For this review, take the finished solid that the model builds, in its own axes (mm). A direction names the side the tool comes from. Round coordinates to 2 decimals unless told otherwise and drop trailing zeros. Write each loop counter-clockwise with the first axis right and the second up, starting at its lowest first coordinate (ties: lowest second). Pieces come first, ordered by that corner, then holes. Notation, with made-up numbers: (-36, 80) -> (-1, 80) arc R17 cw to (-1, 96) -> close; hole circle Ø1 at (86.5, 23.25). An arc over 180 degrees is marked (long way). Answer as CSV lines item,"result". Start each with the question number.
Item 1: Take a section at D-D on y = -2.5. Give the boundary of the cut face in (x, z).
Item 2: For pin 1 Ø1.5 at (y, z) = (-1, -35) entering from +X; pin 2 Ø4 at (y, z) = (2.5, -1) entering from -X; pin 3 Ø6 at (x, z) = (-0.5, -7.5) entering from -Y, all flat-tipped, find the tip position at first contact; note any pin that passes through.
Item 3: Take a section at B-B on z = -32. Give the boundary of the cut face in (x, y).
Item 4: Take a section at A-A on y = 0. Give the boundary of the cut face in (x, z), then the cut area to 3 significant figures.
Item 5: Wall thickness on probe 1 along Z at (x, y) = (2.25, 2.75); probe 2 along Y at (x, z) = (0, -8.5); probe 3 along Z at (x, y) = (1, 1): over which ranges is each line inside the solid? List them lowest first. Write a range as from..to.
Item 6: Mouldability with a two-part tool opening along Y and no side actions: class faces 1 (the flat face through (0, 0, -40)), 2 (the cylindrical face through (-3, 0, -20)), 3 (the flat face through (-1.8, -2.4, 6)) as +Y half, -Y half, draft (parallel to the pull), parting line (faces both ways), or undercut.
Item 7: Take a section at C-C on x = 3.75. Give the boundary of the cut face in (y, z).
Item 8: Machinability: for faces 4 (the cylindrical face through (-1.08, -4.88, 3.94)), 5 (the flat face through (-0.1, -3.3, 0)), 6 (the flat face through (-1.18, 2.76, 6.03)), which of the approach directions +Z, -Z, +X, -X, +Y, -Y give a long, thin tool a straight path to every point of the face, cutting with its end or side? Answer none if there is none.
```python
from build123d import *

# Parameters (mm, degrees)
SZKIC1_R                    = 5
DODANIE_WYCI_GNI_CIE1_DEPTH = 8
SZKIC2_R                    = 3
DODANIE_WYCI_GNI_CIE2_DEPTH = 40
WYTNIJ_WYCI_GNI_CIE1_DEPTH  = 4


with BuildPart() as part:
    # Szkic1 → Dodanie-wyciągnięcie1 (new body)
    with BuildSketch(Plane.XY):
        Circle(SZKIC1_R)
    extrude(amount=DODANIE_WYCI_GNI_CIE1_DEPTH)

    # Szkic2 → Dodanie-wyciągnięcie2 (add)
    with BuildSketch(Plane.XY):
        Circle(SZKIC2_R)
    extrude(amount=-DODANIE_WYCI_GNI_CIE2_DEPTH)

    # Szkic3 → Wytnij-wyciągnięcie1 (cut)
    with BuildSketch(Plane.XY.offset(8)):
        Polygon((2.791473495, -2.051261985), (3.172181736, 1.391855968), (0.380708241, 3.443117953), (-2.791473495, 2.051261985), (-3.172181736, -1.391855968), (-0.380708241, -3.443117953), align=None)
    extrude(amount=-WYTNIJ_WYCI_GNI_CIE1_DEPTH, mode=Mode.SUBTRACT)


solid = part.part
```
Output values:
1,outline,"(-4.33, 0) -> (-1.66, 0) -> (-1.66, -40) -> (1.66, -40) -> (1.66, 0) -> (4.33, 0) -> (4.33, 8) -> (1.77, 8) -> (1.77, 4) -> (-1.66, 4) -> (-1.66, 8) -> (-4.33, 8) -> close"
2,pin 1,"stops at x = 2.99"
2,pin 2,"stops at x = -4.94"
2,pin 3,"stops at y = -3"
3,outline,"circle Ø6 at (0, 0)"
4,outline,"(-5, 0) -> (-3, 0) -> (-3, -40) -> (3, -40) -> (3, 0) -> (5, 0) -> (5, 8) -> (3.02, 8) -> (3.02, 4) -> (-3.02, 4) -> (-3.02, 8) -> (-5, 8) -> close"
4,area,"296 mm^2"
5,probe 1,"z = 0..8"
5,probe 2,"y = -3..3"
5,probe 3,"z = -40..4"
6,face 1,"draft"
6,face 2,"parting line"
6,face 3,"undercut"
7,outline,"(-3.31, 0) -> (3.31, 0) -> (3.31, 8) -> (-3.31, 8) -> close"
8,face 4,"+Z, -Z"
8,face 5,"-Z"
8,face 6,"+Z"
